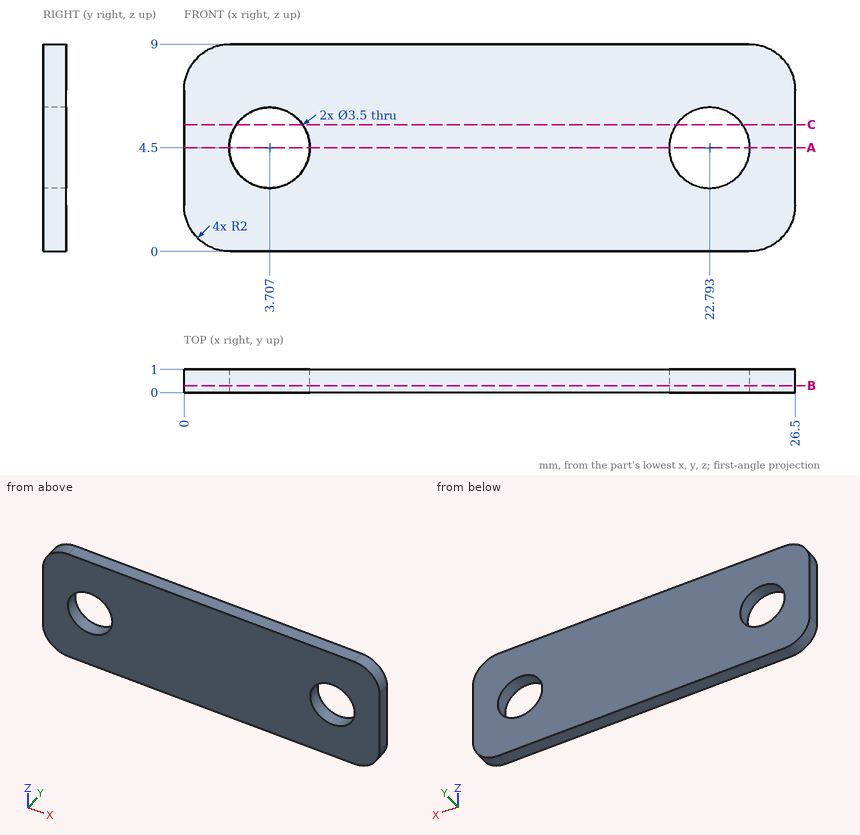
Can you work these out from the drawing? Everything is in mm from the part's minimum corner. Give positions to 0.01 mm unless a question says otherwise; leave off trailing zeros. Loops run counter-clockwise (first coordinate to the right, second up) from the corner with the lowest first, then second, coordinate; pieces in that order, holes last. Notation, with made-up numbers: M 7.25,11 L 19.25,11 A28 ccw 19.25,42 Z; hole C -34.5,36 d2. An arc over 180 degrees is marked long. Use CSV: the item, a comma, the result in double quotes. Start each with the question number.
1. For P1, Ø3, axis at x = 22.793, z = 4.5, coming from the +Y side, with a flat end and sliding along its axis, tell me the tip position at first contact or that it passes through.
2. Imagine slicing it at B-B, the plane y = 0.3. Write out the boundary of the cut face in (x, z), plus the area to 3 significant figures.
3. Imagine slicing it at A-A, the plane z = 4.5. Write out the boundary of the cut face in (x, y), plus the area to 3 significant figures.
4. Imagine slicing it at C-C, the plane z = 5.5. Write out the boundary of the cut face in (x, y).
5. If I drill on L1, parallel to X at y = 0.75, z = 3.5; L2, parallel to X at y = 0.45, z = 4.75; L3, parallel to Z at x = 3, y = 0.4, over which ranges is the centre line in solid material (lowest first)?
Response values:
1,P1,"through"
2,outline,"M 0,2 A2 ccw 2,0 L 24.5,0 A2 ccw 26.5,2 L 26.5,7 A2 ccw 24.5,9 L 2,9 A2 ccw 0,7 Z; hole C 3.71,4.5 d3.5; hole C 22.79,4.5 d3.5"
2,area,"216 mm^2"
3,outline,"M 0,0 L 1.96,0 L 1.96,1 L 0,1 Z; M 5.46,0 L 21.04,0 L 21.04,1 L 5.46,1 Z; M 24.54,0 L 26.5,0 L 26.5,1 L 24.54,1 Z"
3,area,"19.5 mm^2"
4,outline,"M 0,0 L 2.27,0 L 2.27,1 L 0,1 Z; M 5.14,0 L 21.36,0 L 21.36,1 L 5.14,1 Z; M 24.23,0 L 26.5,0 L 26.5,1 L 24.23,1 Z"
5,L1,"0 to 2.27, 5.14 to 21.36, 24.23 to 26.5"
5,L2,"0 to 1.97, 5.44 to 21.06, 24.53 to 26.5"
5,L3,"0 to 2.9, 6.1 to 9"
